The model under review builds one solid part; all positions refer to its coordinate system, in mm. Face numbers are marked on the shaded views. A direction names the side the tool comes from. Round coordinates to 2 decimals unless told otherwise and drop trailing zeros. Loops run counter-clockwise (first coordinate to the right, second up) from the corner with the lowest first, then second, coordinate; pieces in that order, holes last. Notation, with made-up numbers: M 51.25,34 L 69.25,34 A24 cw 69.25,47 Z; hole C -24,31 d3. An arc over 180 degrees is marked long. Answer as a JSON object with one key per item and string values. Group by question number.
Item 1: To check wall thickness, follow line 1 (Y direction, x = 5.5, z = 25); line 2 (Z direction, x = 3, y = -37.5); line 3 (Y direction, x = 6, z = 20). State the ranges of each line that lie inside material, in increasing order.
Item 2: Consider section A-A (z = 13.5). Give the boundary of the cut face in (x, y).
Item 3: Consider section D-D (z = 40.5). Give the boundary of the cut face in (x, y).
Item 4: Insertion check: P1, Ø5, axis at x = 2, y = -42.5, coming from the -Z side; P2, Ø3.5, axis at y = 79.64, z = 24.5, coming from the +X side; P3, Ø7.5, axis at x = 8, z = 16, coming from the -Y side; P4, Ø1.5, axis at x = 7.5, z = 30.5, coming from the +Y side. Each pin has a flat end and moves straight along its axis. Give the tip position at first contact, or say it passes through.
Item 5: The part is to be moulded in two halves that separate along Y. For the marked faces 5, 6 and 7, say which applies: +Y half, -Y half, draft (parallel to the pull), parting line (faces both ways), or undercut.
Item 6: Consider section B-B (x = 6.5). Give the boundary of the cut face in (y, z), and give its area (3 significant figures).
Item 7: Consider section C-C (y = 11). Give the boundary of the cut face in (x, z), and give its area (3 significant figures).
Item 8: Tool access review of the marked faces 1, 2, 3 and 4: name each direction out of +Z, -Z, +X, -X, +Y, -Y from which nothing blocks a thin tool from reaching the whole face with its end or side.
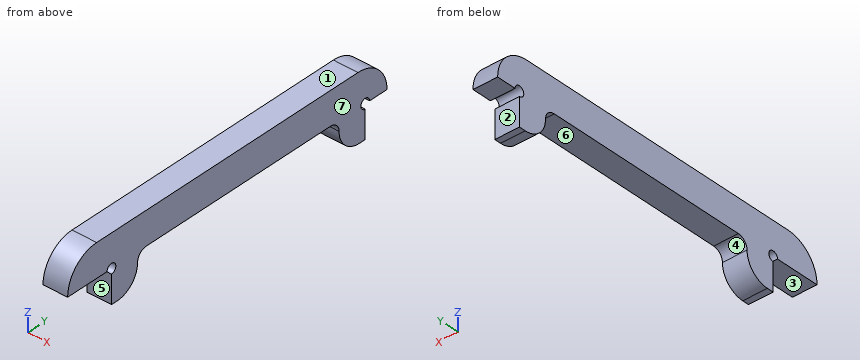
```python
from build123d import *

# Parameters (mm, degrees)
F1_DEPTH = 15


# Not quite as in the source:
# - a feature names something its author has since deleted; it is built from what else it names


with BuildPart() as f1:
    # F0 (on Right) → F1 (new body)
    with BuildSketch(Plane.YZ):
        with BuildLine():
            Line((-15.3621651637, 44.4962902069), (-105.3621651637, 44.4962902069))
            ThreePointArc((-105.3621651637, 44.4962902069), (-119.5043007874, 38.6384258306), (-125.3621651637, 24.4962902069))
            Line((-125.3621651637, 24.4962902069), (-98.1621651637, 24.4962902069))
            ThreePointArc((-98.1621651637, 24.4962902069), (-93.0408448201, 26.6176105505), (-95.1621651637, 21.4962902069))
            Line((-95.1621651637, 21.4962902069), (-95.1621651637, 4.4962902069))
            Line((-95.1621651637, 4.4962902069), (-91.1621651637, 4.4962902069))
            ThreePointArc((-91.1621651637, 4.4962902069), (-81.2626702271, 8.5967952703), (-77.1621651637, 18.4962902069))
            ThreePointArc((-77.1621651637, 18.4962902069), (-75.4048058508, 22.738930894), (-71.1621651637, 24.4962902069))
            Line((-71.1621651637, 24.4962902069), (-15.3621651637, 24.4962902069))
            Line((-15.3621651637, 24.4962902069), (40.4378348363, 24.4962902069))
            Line((40.4378348363, 24.4962902069), (55.6378348363, 24.4962902069))
            ThreePointArc((55.6378348363, 24.4962902069), (59.8804755234, 22.738930894), (61.6378348363, 18.4962902069))
            ThreePointArc((61.6378348363, 18.4962902069), (65.7383398997, 8.5967952703), (75.6378348363, 4.4962902069))
            Line((75.6378348363, 4.4962902069), (79.6378348363, 4.4962902069))
            Line((79.6378348363, 4.4962902069), (79.6378348363, 21.4962902069))
            ThreePointArc((79.6378348363, 21.4962902069), (77.5165144927, 26.6176105505), (82.6378348363, 24.4962902069))
            Line((82.6378348363, 24.4962902069), (94.6378348363, 24.4962902069))
            ThreePointArc((94.6378348363, 24.4962902069), (88.77997046, 38.6384258306), (74.6378348363, 44.4962902069))
            Line((74.6378348363, 44.4962902069), (-15.3621651637, 44.4962902069))
        make_face()
    extrude(amount=F1_DEPTH)


solid = f1.part
```
Geometry results:
{
 "1": {"line 1": "y = -125.36 to -98.12, -92.2 to 76.68, 82.6 to 94.63", "line 2": "z = 24.5 to 44.5", "line 3": "y = -95.16 to -76.97, 61.45 to 79.64"},
 "2": {"outline": "M 0,-95.16 L 15,-95.16 L 15,-78.08 L 0,-78.08 Z; M 0,62.56 L 15,62.56 L 15,79.64 L 0,79.64 Z"},
 "3": {"outline": "M 0,-117.36 L 15,-117.36 L 15,86.63 L 0,86.63 Z"},
 "4": {"P1": "stops at z = 24.5", "P2": "passes through", "P3": "stops at y = -95.16", "P4": "stops at y = 93.94"},
 "5": {"face 5": "-Y half", "face 6": "undercut", "face 7": "draft"},
 "6": {"outline": "M -125.36,24.5 L -98.16,24.5 A3 cw long -95.16,21.5 L -95.16,4.5 L -91.16,4.5 A14 ccw -77.16,18.5 A6 cw -71.16,24.5 L 55.64,24.5 A6 cw 61.64,18.5 A14 ccw 75.64,4.5 L 79.64,4.5 L 79.64,21.5 A3 cw long 82.64,24.5 L 94.64,24.5 A20 ccw 74.64,44.5 L -105.36,44.5 A20 ccw Z", "area": "4,840 mm^2"},
 "7": {"outline": "M 0,24.5 L 15,24.5 L 15,44.5 L 0,44.5 Z", "area": "300 mm^2"},
 "8": {"face 1": "+Z, +X, -X, +Y, -Y", "face 2": "-Z, +X, -X, +Y", "face 3": "-Z, +X, -X, -Y", "face 4": "-Z, +X, -X"}
}
